Work out the finished part from the listing and answer in its coordinate system (mm). A direction names the side the tool comes from. Round coordinates to 2 decimals unless told otherwise and drop trailing zeros. Order: outer loops, then holes, each group sorted by start corner. A loop starts at its lowest first (then second) coordinate and runs counter-clockwise, first axis right, second up. Notation, with made-up numbers: (78, -27.75) - (120, -27.75) arc R22 ccw to (120, -8.75) - close; hole circle Ø3 at (69, 31.5). An arc over 180 degrees is marked (long way). Answer in a Markdown table with one row per item.
from build123d import *

# Parameters (mm, degrees)
SKETCH1_W                     = 7.5
SKETCH1_H                     = 17.5
BOSS_EXTRUDE1_DEPTH           = 3.5
SKETCH2_W                     = 5.5
SKETCH2_H                     = 15.5
CUT_EXTRUDE1_DEPTH            = 2.5
SKETCH3_R                     = 1.5
GRIN_HOLE_DEPTH               = 2
SKETCH6_R                     = 0.5953125
CORNER_DIVOT_DEPTH            = 2.5
SKETCH7_R                     = 0.79375
MAGNET_HOLES_DEPTH            = 2
BOSS_EXTRUDE2_DEPTH           = 3.5
SKETCH14_W                    = 5.965258944
SKETCH14_H                    = 5.132960456
SET_SCREW_EXTENSION_DEPTH     = 0.75
TAP_DRILL_FOR_0_80_TAP1_D     = 1.19126
TAP_DRILL_FOR_0_80_TAP1_DEPTH = 7.11
TAP_DRILL_FOR_0_80_TAP1_TIP   = 0.357890611
DIAGONAL_CUT_DEPTH            = 5
SKETCH16_W                    = 1
SKETCH16_H                    = 15.5
VERTICAL_CUT_DEPTH            = 3


with BuildPart() as part:
    # Sketch1 → Boss-Extrude1 (new body)
    with BuildSketch(Plane(origin=(0, 0, 0), x_dir=(1, 0, 0), z_dir=(0, 1, 0))):
        Rectangle(SKETCH1_W, SKETCH1_H)
    extrude(amount=BOSS_EXTRUDE1_DEPTH)

    # Sketch2 → Cut-Extrude1 (cut)
    with BuildSketch(Plane(origin=(0, 3.5, 0), x_dir=(1, 0, 0), z_dir=(0, 1, 0))):
        Rectangle(SKETCH2_W, SKETCH2_H)
    extrude(amount=-CUT_EXTRUDE1_DEPTH, mode=Mode.SUBTRACT)

    # Sketch3 → GRIN Hole (cut, through all)
    with BuildSketch(Plane(origin=(0, 1, 0), x_dir=(1, 0, 0), z_dir=(0, 1, 0))):
        with Locations((-0.25, -4.75)):
            Circle(SKETCH3_R)
    extrude(amount=-GRIN_HOLE_DEPTH, mode=Mode.SUBTRACT)

    # Sketch6 → Corner divot (cut)
    with BuildSketch(Plane(origin=(0, 3.5, 0), x_dir=(1, 0, 0), z_dir=(0, 1, 0))):
        with Locations((2.329050494, -7.329050494)):
            Circle(SKETCH6_R)
    extrude(amount=-CORNER_DIVOT_DEPTH, mode=Mode.SUBTRACT)

    # Sketch7 → Magnet Holes (cut, through all)
    with BuildSketch(Plane(origin=(0, 1, 0), x_dir=(1, 0, 0), z_dir=(0, 1, 0))):
        with Locations((-0.25, 2.25)):
            Circle(SKETCH7_R)
        with Locations((-2.125, -6.5)):
            Circle(SKETCH7_R)
        with Locations((1.625, -6.5)):
            Circle(SKETCH7_R)
    extrude(amount=-MAGNET_HOLES_DEPTH, mode=Mode.SUBTRACT)

    # Sketch9 → Boss-Extrude2 (add)
    with BuildSketch(Plane(origin=(0, 3.5, 0), x_dir=(1, 0, 0), z_dir=(0, 1, 0))):
        Polygon((-2.493978672, 9.405385289), (-4.710390263, 8.248873438), (-4.086258113, 7.05274758), (-3.457701518, 7.380725089), (-2.498403119, 7.881281923), (-1.869846523, 8.209259431), align=None)
    extrude(amount=-BOSS_EXTRUDE2_DEPTH)

    # Sketch14 → Set Screw Extension (cut)
    with BuildSketch(Plane(origin=(0, 3.5, 0), x_dir=(1, 0, 0), z_dir=(0, 1, 0))):
        with Locations((-2.75, 7.75)):
            Rectangle(SKETCH14_W, SKETCH14_H)
    extrude(amount=-SET_SCREW_EXTENSION_DEPTH, mode=Mode.SUBTRACT)

    # Tap Drill for #0-80 Tap1
    with Locations(Plane(origin=(-4.391140577, 0, -8.415456236), x_dir=(-0.886564636, 0, 0.46260474), z_dir=(-0.46260474, 0, -0.886564636))):
        with Locations((-0.889902526, 1.875)):
            Hole(TAP_DRILL_FOR_0_80_TAP1_D / 2, depth=TAP_DRILL_FOR_0_80_TAP1_DEPTH)
            with Locations((0, 0, -(TAP_DRILL_FOR_0_80_TAP1_DEPTH + TAP_DRILL_FOR_0_80_TAP1_TIP / 2))):  # 118° drill point
                Cone(0, TAP_DRILL_FOR_0_80_TAP1_D / 2, TAP_DRILL_FOR_0_80_TAP1_TIP, mode=Mode.SUBTRACT)

    # Sketch15 → Diagonal Cut (cut)
    with BuildSketch(Plane(origin=(0, 0, 0), x_dir=(1, 0, 0), z_dir=(0, 1, 0))):
        Polygon((-2.152002093, 9.313235547), (-2.152002093, 7.75), (3.75, -0.208562074), (3.75, 9.313235547), align=None)
    extrude(amount=DIAGONAL_CUT_DEPTH, mode=Mode.SUBTRACT)

    # Sketch16 → Vertical Cut (cut)
    with BuildSketch(Plane(origin=(0, 1, 0), x_dir=(1, 0, 0), z_dir=(0, 1, 0))):
        with Locations((-3.25, 0)):
            Rectangle(SKETCH16_W, SKETCH16_H)
    extrude(amount=VERTICAL_CUT_DEPTH, mode=Mode.SUBTRACT)


solid = part.part
1) Find section B-B, the plane x = -0.25. Give the vertices of the cut face in (y, z), then the cut area to 3 significant figures.
Filled in:
| item | result |
|---|---|
| outline | (0, -5.19) - (1, -5.19) - (1, -3.04) - (0, -3.04) - close; (0, -1.46) - (1, -1.46) - (1, 3.25) - (0, 3.25) - close; (0, 6.25) - (1, 6.25) - (1, 7.75) - (3.5, 7.75) - (3.5, 8.75) - (0, 8.75) - close |
| area | 11.8 mm^2 |
2) The mould has two halves that part along X. Classify faces 6 (the face through (-2.835, 1.647, -8.546)), 7 (the face through (2.75, 2, 3)), 8 (the face through (-3, 2.75, -8)): released by +X, released by -X, zero draft, split by the parting line, or undercut.
Filled in:
| item | result |
|---|---|
| face 6 | undercut |
| face 7 | released by -X |
| face 8 | zero draft |
3) Which of the six approach directions +Z, -Z, +X, -X, +Y, -Y give full straight-line access (tool end or side, diameter ignored) to faces 1 (the face through (2.74, 2.27, 7.76)), 2 (the face through (-0.445, 0.507, 3.263)), 3 (the face through (-2.152, 1, -8)), 4 (the face through (3, 3.5, 6)), 5 (the face through (-1, 2, 7.75))?
Filled in:
| item | result |
|---|---|
| face 1 | +Y |
| face 2 | +Y, -Y |
| face 3 | -Z, +X, +Y, -Y |
| face 4 | +Z, -Z, +X, -X, +Y |
| face 5 | -X, +Y |
4) Find the intervals of material crossed by probe 1 along X at (y, z) = (0.7, 6.5); probe 2 along Z at (x, y) = (-0.25, 0.85); probe 3 along X at (y, z) = (0.25, 4.75), in increasing order. Write a range as from..to.
Filled in:
| item | result |
|---|---|
| probe 1 | x = -3.75..-2.92, -1.33..0.83, 2.42..3.75 |
| probe 2 | z = -5.19..-3.04, -1.46..3.25, 6.25..8.75 |
| probe 3 | x = -3.75..-1.75, 1.25..3.75 |
5) Find section D-D, the plane x = 1.5. Give the vertices of the cut face in (y, z), then the cut area to 3 significant figures.
Filled in:
| item | result |
|---|---|
| outline | (0, -2.83) - (1, -2.83) - (1, 5.72) - (0, 5.72) - close; (0, 7.28) - (1, 7.28) - (1, 7.75) - (3.5, 7.75) - (3.5, 8.75) - (0, 8.75) - close |
| area | 12.5 mm^2 |
6) Find section C-C, the plane y = 2.15. Give the vertices of the cut face in (x, z), then the cut area to 3 significant figures.
Filled in:
| item | result |
|---|---|
| outline | (-4.71, -8.25) - (-4.07, -8.58) - (-3.64, -7.75) - (-3.75, -7.75) - (-3.75, -7.23) - (-4.09, -7.05) - close; (-3.75, 7.75) - (1.91, 7.75) arc R0.6 cw to (2.75, 6.91) - (2.75, -1.14) - (3.75, 0.21) - (3.75, 8.75) - (-3.75, 8.75) - close; (-3.13, -9.07) - (-2.49, -9.41) - (-2.15, -8.75) - (-2.15, -7.75) - (-2.44, -7.75) - close |
| area | 17.3 mm^2 |
7) Find section A-A, the plane z = 4.75. Give the vertices of the cut face in (x, y), then the cut area to 3 significant figures.
Filled in:
| item | result |
|---|---|
| outline | (-3.75, 0) - (-1.75, 0) - (-1.75, 1) - (-3.75, 1) - close; (1.25, 0) - (3.75, 0) - (3.75, 3.5) - (2.75, 3.5) - (2.75, 1) - (1.25, 1) - close |
| area | 7.00 mm^2 |
8) Each of these flat-tipped pins is pushed along its axis until it touches: pin 1 (0.8 mm diameter, centred on x = 0.5, y = 2, fed in from -Z); pin 2 (1.1 mm diameter, centred on y = 1, z = -8.5, fed in from +X); pin 3 (1.8 mm diameter, centred on y = 2.5, z = 0.5, fed in from -X). Where does it stop, or does it pass through?
Filled in:
| item | result |
|---|---|
| pin 1 | stops at z = 7.75 |
| pin 2 | stops at x = -2.15 |
| pin 3 | stops at x = 2.75 |
